Could you check a few things on this model? Use its own coordinates, in mm. Face numbers are marked on the shaded views. A direction names the side the tool comes from. Round coordinates to 2 decimals unless told otherwise and drop trailing zeros. Order: outer loops, then holes, each group sorted by start corner. A loop starts at its lowest first (then second) coordinate and runs counter-clockwise, first axis right, second up. Notation, with made-up numbers: (-21, -38.75) - (17, -38.75) arc R19 cw to (17, -8.75) - close; hole circle Ø11 at (-33.5, 15). An arc over 180 degrees is marked (long way). Return JSON: item names as keys, results as strings. Group by question number.
from build123d import *

# Parameters (mm, degrees)
SKETCH1_R                    = 42.799
SKETCH1_R_2                  = 23.8125
BOSS_EXTRUDE1_DEPTH          = 15.748
SKETCH2_R                    = 25.527
CUT_EXTRUDE1_DEPTH           = 10.033
CHAMFER1_SIZE                = 0.762
SKETCH3_R                    = 4.2164
CUT_EXTRUDE2_DEPTH           = 16.748
CHAMFER2_SIZE                = 0.381
CIRPATTERN1_COUNT            = 8
CHAMFER2_OF_CIRPATTERN1_SIZE = 0.381
CUT_EXTRUDE3_DEPTH           = 0.79375


with BuildPart() as part:
    # Sketch1 → Boss-Extrude1 (new body)
    with BuildSketch(Plane(origin=(0, 0, 0), x_dir=(1, 0, 0), z_dir=(0, 1, 0))):
        Circle(SKETCH1_R)
        Circle(SKETCH1_R_2, mode=Mode.SUBTRACT)
    extrude(amount=BOSS_EXTRUDE1_DEPTH)

    # Sketch2 → Cut-Extrude1 (cut)
    with BuildSketch(Plane(origin=(0, 15.748, 0), x_dir=(-1, 0, 0), z_dir=(0, 1, 0))):
        Circle(SKETCH2_R)
    extrude(amount=-CUT_EXTRUDE1_DEPTH, mode=Mode.SUBTRACT)

    # Chamfer1
    chamfer1_edges = [part.edges().sort_by_distance(p)[0] for p in [
        (25.527, 15.748, 0),
        (-42.799, 0, 0),
        (-42.799, 15.748, 0),
    ]]
    chamfer(chamfer1_edges, length=CHAMFER1_SIZE)

    # Sketch5 → Cut-Revolve1 (revolve, cut)
    with BuildSketch(Plane(origin=(0, 0, 0), x_dir=(1, 0, 0), z_dir=(0, 0, -1))):
        Polygon((0, 0), (-30.9499, 0), (-30.9499, -1.75514), (-27.94, -0.6604), (-27.94, -1.27), (0, -1.27), align=None)
    revolve(axis=Axis((0, 15.748, 0), (0, -1, 0)), mode=Mode.SUBTRACT)

    # Sketch3 → Cut-Extrude2 (cut, through all)
    with BuildSketch(Plane.XZ):
        with Locations((-13.851226834, 33.439819679)):
            Circle(SKETCH3_R)
    cut_extrude2 = extrude(amount=-CUT_EXTRUDE2_DEPTH, mode=Mode.SUBTRACT)

    # Chamfer2
    chamfer2_edges = [part.edges().sort_by_distance(p)[0] for p in [
        (-18.067626834, 15.748, 33.439819679),
        (-18.067626834, 0, 33.439819679),
    ]]
    chamfer(chamfer2_edges, length=CHAMFER2_SIZE)

    # CirPattern1: Cut-Extrude2 ×8 about axis
    cirpattern1_axis = Axis((0, 0, 0), (0, 1, 0))
    for i in range(1, CIRPATTERN1_COUNT):
        add(cut_extrude2.rotate(cirpattern1_axis, i * 360 / CIRPATTERN1_COUNT), mode=Mode.SUBTRACT)

    # Chamfer2 of CirPattern1
    chamfer2_of_cirpattern1_edges = [part.edges().sort_by_distance(p)[0] for p in [
        (10.869781802, 15.748, 36.421264711),
        (10.869781802, 0, 36.421264711),
        (33.439819679, 15.748, 18.067626834),
        (33.439819679, 0, 18.067626834),
        (36.421264711, 15.748, -10.869781802),
        (36.421264711, 0, -10.869781802),
        (18.067626834, 15.748, -33.439819679),
        (18.067626834, 0, -33.439819679),
        (-10.869781802, 15.748, -36.421264711),
        (-10.869781802, 0, -36.421264711),
        (-33.439819679, 15.748, -18.067626834),
        (-33.439819679, 0, -18.067626834),
        (-36.421264711, 15.748, 10.869781802),
        (-36.421264711, 0, 10.869781802),
    ]]
    chamfer(chamfer2_of_cirpattern1_edges, length=CHAMFER2_OF_CIRPATTERN1_SIZE)

    # Sketch6 → Cut-Extrude3 (cut, symmetric)
    with BuildSketch(Plane.XY):
        Polygon((-42.799, 1.587408258), (-42.799, -0.655592288), (-30.127480656, -0.655592288), (-30.127480656, 0.923322069), align=None)
        Polygon((30.127480656, 0.923322069), (42.799, 1.587408258), (42.799, -0.655592288), (30.127480656, -0.655592288), align=None)
    extrude(amount=CUT_EXTRUDE3_DEPTH, both=True, mode=Mode.SUBTRACT)


solid = part.part
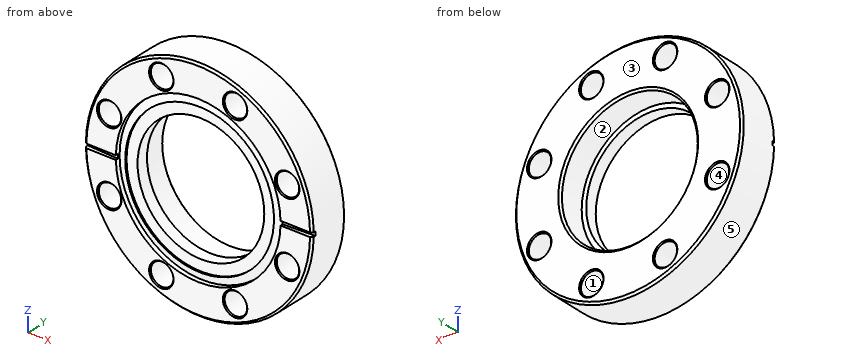
1) For the marked faces 1 and 2, which set-ups out of +Z, -Z, +X, -X, +Y, -Y let a thin tool reach every point of the face, with its end or its side?
2) Will these pins go through, and if not, where does the flat tip stop? pin 1 (1.5 mm diameter, centred on x = -19.5, y = 9.5, fed in from +Z); pin 2 (1.3 mm diameter, centred on x = 34, y = 0.5, fed in from -Z); pin 3 (2 mm diameter, centred on x = 21.5, y = 9, fed in from +Z).
3) We'd pull the mould along X, two halves only. Please class the marked faces 3, 4 and 5: +X half, -X half, draft (parallel to the pull), parting line (faces both ways), or undercut.
4) I want a section at A-A, the plane x = 0. List the corners of the cut face in (y, z) for me (1 decimal).
5) I want a section at B-B, the plane y = 2.75. Give the number of separate pieces and of enclosed holes in the cut face, plus the area to 3 significant figures.
6) If I drill on line 1 along Z through (x, y) = (15.5, 6); line 2 along X through (y, z) = (4.75, 14); line 3 along X through (y, z) = (12.75, 12.5), over which ranges is the centre line in solid material (lowest first)? Write a range as from..to.
Outcome:
{
 "1": {"face 1": "+Y, -Y", "face 2": "+Y"},
 "2": {"pin 1": "z = 38.47", "pin 2": "z = -26.76", "pin 3": "z = 37.57"},
 "3": {"face 3": "draft", "face 4": "undercut", "face 5": "parting line"},
 "4": {"outline": "(0, -42) - (0.8, -42.8) - (15, -42.8) - (15.7, -42) - (15.7, -26.3) - (15, -25.5) - (5.7, -25.5) - (5.7, -23.8) - (1.3, -23.8) - (1.3, -27.9) - (0.7, -27.9) - (1.8, -30.9) - (0, -30.9) - close; (0, 30.9) - (1.8, 30.9) - (0.7, 27.9) - (1.3, 27.9) - (1.3, 23.8) - (5.7, 23.8) - (5.7, 25.5) - (15, 25.5) - (15.7, 26.3) - (15.7, 42) - (15, 42.8) - (0.8, 42.8) - (0, 42) - close"},
 "5": {"separate pieces": "1", "enclosed holes": "9", "area": "3,530 mm^2"},
 "6": {"line 1": "-39.89..-37.32, -29.56..-20.28, 20.28..29.56, 37.32..39.89", "line 2": "-40.44..-37.65, -29.23..-19.26, 19.26..29.23, 37.65..40.44", "line 3": "-40.93..-37.43, -29.45..-22.26, 22.26..29.45, 37.43..40.93"}
}
